from build123d import *

# Parameters (mm, degrees)
F1_DEPTH = 40
F2_R     = 2.5
F3_DEPTH = 25
F4_R     = 2.5
F5_DEPTH = 25


with BuildPart() as f1:
    # F0 (on Front) → F1 (new body, symmetric)
    with BuildSketch(Plane.XZ):
        Polygon((-80, 2.5), (-80, 0), (0, 0), (0, 80), (-2.5, 80), (-2.5, 2.5), align=None)
    extrude(amount=F1_DEPTH, both=True)

    # F2 (on face) → F3 (cut)
    with BuildSketch(Plane(origin=(-2.5, 0, 0), x_dir=(0, -1, 0), z_dir=(-1, 0, 0))):
        with Locations((0, 41.25)):
            Circle(F2_R)
        with Locations((-34, 8.5)):
            Circle(F2_R)
        with Locations((-34, 74)):
            Circle(F2_R)
        with Locations((34, 74)):
            Circle(F2_R)
        with Locations((34, 8.5)):
            Circle(F2_R)
    extrude(amount=-F3_DEPTH, mode=Mode.SUBTRACT)

    # F4 (on face) → F5 (cut)
    with BuildSketch(Plane.XY.offset(2.5)):
        with Locations((-74, 0)):
            Circle(F4_R)
        with Locations((-41.25, 34)):
            Circle(F4_R)
        with Locations((-41.25, -34)):
            Circle(F4_R)
        with Locations((-8.5, 0)):
            Circle(F4_R)
    extrude(amount=-F5_DEPTH, mode=Mode.SUBTRACT)


solid = f1.part
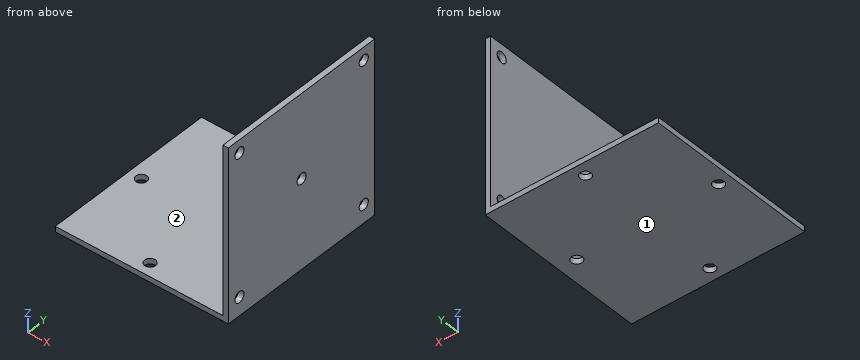
Input: part model. Units: mm. Frame: model coordinates. Face numbers are marked on the shaded views. A direction names the side the tool comes from. Round coordinates to 2 decimals unless told otherwise and drop trailing zeros. Write each loop counter-clockwise with the first axis right and the second up, starting at its lowest first coordinate (ties: lowest second). Pieces come first, ordered by that corner, then holes.
1) Cut plane C-C (y = 34). Return the cut outline in (x, z), then the cut area to 3 significant figures.
2) Contact query for flat-ended pins moving along their axis: P1, Ø3, axis at y = 34, z = 74, coming from the -X side; P2, Ø1.5, axis at y = 6.5, z = 68, coming from the +X side; P3, Ø12, axis at y = -19.5, z = 52.5, coming from the -X side; P4, Ø2, axis at x = -36, y = -12.5, coming from the +Z side. Output: stop coordinate, or through.
3) Cut plane A-A (z = 41.25). Return the cut outline in (x, y), then the cut area to 4 significant figures.
4) Cut plane D-D (x = -41.25). Return the cut outline in (y, z).
5) Reachability of the marked faces 1 and 2 from +Z, -Z, +X, -X, +Y, -Y: full face, straight path, thin tool, end or side. Return the list, or none.
6) Cut plane B-B (z = 74). Return the cut outline in (x, y), then the cut area to 3 significant figures.
7) Ray query, L1, parallel to Z at x = -1, y = 34; L2, parallel to Z at x = -1, y = 0; L3, parallel to X at y = -7, z = 25. Return the intervals inside material, ascending.
Geometry says:
1. outline: (-80, 0) - (-43.75, 0) - (-43.75, 2.5) - (-80, 2.5) - close; (-38.75, 0) - (0, 0) - (0, 6) - (-2.5, 6) - (-2.5, 2.5) - (-38.75, 2.5) - close; (-2.5, 11) - (0, 11) - (0, 71.5) - (-2.5, 71.5) - close; (-2.5, 76.5) - (0, 76.5) - (0, 80) - (-2.5, 80) - close
1. area: 356 mm2
2. P1: passes through
2. P2: stops at x = 0
2. P3: stops at x = -2.5
2. P4: stops at z = 2.5
3. outline: (-2.5, -40) - (0, -40) - (0, -2.5) - (-2.5, -2.5) - close; (-2.5, 2.5) - (0, 2.5) - (0, 40) - (-2.5, 40) - close
3. area: 187.5 mm2
4. outline: (-40, 0) - (-36.5, 0) - (-36.5, 2.5) - (-40, 2.5) - close; (-31.5, 0) - (31.5, 0) - (31.5, 2.5) - (-31.5, 2.5) - close; (36.5, 0) - (40, 0) - (40, 2.5) - (36.5, 2.5) - close
5. face 1: -Z, +X, -X, +Y, -Y
5. face 2: +Z, -X, +Y, -Y
6. outline: (-2.5, -40) - (0, -40) - (0, -36.5) - (-2.5, -36.5) - close; (-2.5, -31.5) - (0, -31.5) - (0, 31.5) - (-2.5, 31.5) - close; (-2.5, 36.5) - (0, 36.5) - (0, 40) - (-2.5, 40) - close
6. area: 175 mm2
7. L1: z = 0 to 6, 11 to 71.5, 76.5 to 80
7. L2: z = 0 to 38.75, 43.75 to 80
7. L3: x = -2.5 to 0
